from build123d import *

# Parameters (mm, degrees)
SKETCH1_R             = 95
BOSS_EXTRUDE1_DEPTH   = 27
SKETCH2_R             = 17.5
CUT_EXTRUDE1_DEPTH    = 138.03649149
SKETCH3_R             = 2.368500587
CUT_EXTRUDE2_DEPTH    = 16.795881
CIRPATTERN1_START     = 10.20411943
CIRPATTERN1_OUTLINE_R = 2.368500587
CIRPATTERN1_DEPTH     = 16.79588057


# Read off the part's stored shape, not the designer's step: CirPattern1
with BuildPart() as part:
    # Sketch1 → Boss-Extrude1 (new body)
    with BuildSketch(Plane(origin=(0, 0, 0), x_dir=(1, 0, 0), z_dir=(0, 1, 0))):
        with Locations(Location((0, 0, 0), (0, 0, 270))):
            Circle(SKETCH1_R)
    extrude(amount=BOSS_EXTRUDE1_DEPTH)

    # Sketch2 → Cut-Extrude1 (cut, through all)
    with BuildSketch(Plane(origin=(0, 0, 0), x_dir=(1, 0, 0), z_dir=(0, 1, 0))):
        with Locations(Location((0, 0, 0), (0, 0, 270))):
            Circle(SKETCH2_R)
    extrude(amount=CUT_EXTRUDE1_DEPTH, mode=Mode.SUBTRACT)

    # Sketch3 → Cut-Extrude2 (cut)
    with BuildSketch(Plane(origin=(0, 27, 0), x_dir=(1, 0, 0), z_dir=(0, 1, 0))):
        with Locations(Location((-38.023879586, 0, 0), (0, 0, 270))):
            Circle(SKETCH3_R)
    extrude(amount=-CUT_EXTRUDE2_DEPTH, mode=Mode.SUBTRACT)

    # CirPattern1 outline → CirPattern1 (cut)
    with BuildSketch(Plane(origin=(0, 0, 0), x_dir=(1, 0, 0), z_dir=(0, 1, 0)).offset(CIRPATTERN1_START)):
        with Locations((-19.011939793, -32.929645672)):
            Circle(CIRPATTERN1_OUTLINE_R)
        with Locations((19.011939793, -32.929645672)):
            Circle(CIRPATTERN1_OUTLINE_R)
        with Locations((38.023879586, 0)):
            Circle(CIRPATTERN1_OUTLINE_R)
        with Locations((19.011939793, 32.929645672)):
            Circle(CIRPATTERN1_OUTLINE_R)
        with Locations((-19.011939793, 32.929645672)):
            Circle(CIRPATTERN1_OUTLINE_R)
    extrude(amount=CIRPATTERN1_DEPTH, mode=Mode.SUBTRACT)


solid = part.part
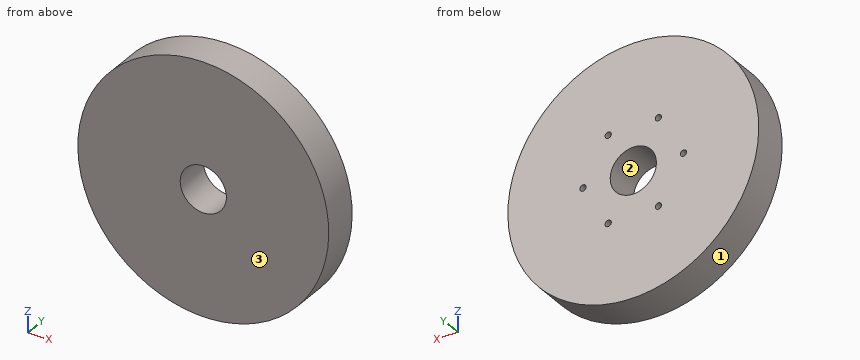
Read the model definition and answer for the solid it produces. Units are mm, in the model's axes. Face numbers are marked on the shaded views. Give positions to 0.01 mm unless a question says otherwise; leave off trailing zeros. Loops run counter-clockwise (first coordinate to the right, second up) from the corner with the lowest first, then second, coordinate; pieces in that order, holes last. Notation, with made-up numbers: (-29, 75) - (-23, 75) arc R21 ccw to (-23, 98) - close; hole circle Ø10 at (40.5, 63.5). An arc over 180 degrees is marked (long way). Answer as CSV lines item,"result". Start each with the question number.
1) Find section A-A (x = 0). Write down the section's boundary in (y, z), then the cut area to 4 significant figures.
2) Each of these flat-tipped pins is pushed along its axis until it touches: pin 1 Ø2 at (x, y) = (-43, 24) entering from -Z; pin 2 Ø2.5 at (x, z) = (19.5, -33.5) entering from +Y; pin 3 Ø2.5 at (x, z) = (-18, 34) entering from +Y; pin 4 Ø10 at (y, z) = (16, 74.5) entering from +X. Where does it stop, or does it pass through?
3) Find section C-C (y = 14.75). Write down the section's boundary in (x, z), then the cut area to 3 significant figures.
4) Determine the mould class of the marked faces 1, 2 and 3 for opening direction X: released by +X, released by -X, zero draft, split by the parting line, or undercut.
5) Straight lines are drawn through the part: L1, parallel to X at y = 18, z = 0; L2, parallel to X at y = 7, z = 0; L3, parallel to Z at x = 8.5, y = 26. For each, find the intervals that lie inside material, in ascending order. Write a range as from..to.
6) Find section B-B (z = 0). Write down the section's boundary in (x, y).
7) Find section D-D (y = 2.75). Write down the section's boundary in (x, z), then the cut area to 3 significant figures.
Findings below:
1,outline,"(0, -95) - (27, -95) - (27, -17.5) - (0, -17.5) - close; (0, 17.5) - (27, 17.5) - (27, 95) - (0, 95) - close"
1,area,"4,185 mm^2"
2,pin 1,"z = -85.21"
2,pin 2,"y = 10.2"
2,pin 3,"y = 27"
2,pin 4,"x = 64.77"
3,outline,"circle Ø190 at (0, 0); hole circle Ø4.74 at (-38.02, 0); hole circle Ø4.74 at (-19.01, -32.93); hole circle Ø4.74 at (-19.01, 32.93); hole circle Ø35 at (0, 0); hole circle Ø4.74 at (19.01, -32.93); hole circle Ø4.74 at (19.01, 32.93); hole circle Ø4.74 at (38.02, 0)"
3,area,"27,300 mm^2"
4,face 1,"split by the parting line"
4,face 2,"undercut"
4,face 3,"zero draft"
5,L1,"-95..-40.39, -35.66..-17.5, 17.5..35.66, 40.39..95"
5,L2,"-95..-17.5, 17.5..95"
5,L3,"-94.62..-15.3, 15.3..94.62"
6,outline,"(-95, 0) - (-17.5, 0) - (-17.5, 27) - (-35.66, 27) - (-35.66, 10.2) - (-40.39, 10.2) - (-40.39, 27) - (-95, 27) - close; (17.5, 0) - (95, 0) - (95, 27) - (40.39, 27) - (40.39, 10.2) - (35.66, 10.2) - (35.66, 27) - (17.5, 27) - close"
7,outline,"circle Ø190 at (0, 0); hole circle Ø35 at (0, 0)"
7,area,"27,400 mm^2"
